The listing builds one solid part. Answer for the finished solid, in the listing's coordinates (mm). A direction names the side the tool comes from. Give positions to 0.01 mm unless a question says otherwise; leave off trailing zeros. Order: outer loops, then holes, each group sorted by start corner. A loop starts at its lowest first (then second) coordinate and runs counter-clockwise, first axis right, second up. Notation, with made-up numbers: (50, -3) - (82, -3) arc R36 ccw to (82, 31) - close; hole circle Ø4 at (89, 12.5). An arc over 180 degrees is marked (long way). Answer as a JSON object with one key per item and string values. Group by question number.
Q1. For faces 1 (the face through (-5.86, 93.18, -11.4)), 2 (the face through (-6.007, 48.669, -10.924)), 3 (the face through (11, 62.5, -30)), determine the directions among +Z, -Z, +X, -X, +Y, -Y from which every point of the face is accessible in a straight line to the end or side of a thin tool.
Q2. A cutting plane is placed at A-A, the plane y = 65. Give the vertices of the cut face in (x, z).
Q3. A cutting plane is placed at B-B, the plane y = 24. Give the vertices of the cut face in (x, z), and give its area (3 significant figures).
Q4. The mould has two halves that part along X. Classify faces 4 (the face through (18.2, 55, -20.1)), 5 (the face through (-5.86, -2.88, -11.4)), 6 (the face through (13.78, 124.33, -23.65)), 7 (the face through (-0.46, 8.52, -40.49)): released by +X, released by -X, zero draft, split by the parting line, or undercut.
Q5. Given pin 1 (3 mm diameter, centred on y = 87, z = -32, fed in from +X); pin 2 (4 mm diameter, centred on y = 43, z = -24.5, fed in from +X); pin 3 (2 mm diameter, centred on x = 13.86, z = -38, fed in from +Y), each flat-ended and moving along its own axis, determine where each tip first touches the part or whether it passes through.
Q6. Consider line 1 (X direction, y = 127.75, z = -46); line 2 (X direction, y = -2, z = -30); line 3 (X direction, y = 121.25, z = -22). Determine where each line is inside the solid, lowest interval first.
from build123d import *

# Parameters (mm, degrees)
SKETCH6_W                     = 2.15
SKETCH6_H                     = 180.5
M4_CLEARANCE_HOLE2_AT_2_COUNT = 2
M4_CLEARANCE_HOLE2_AT_2_PITCH = 16
M4_CLEARANCE_HOLE2_AT_3_COUNT = 2
M4_CLEARANCE_HOLE2_AT_3_PITCH = 27.712812921
M4_CLEARANCE_HOLE2_AT_4_COUNT = 2
M4_CLEARANCE_HOLE2_AT_4_PITCH = 32
M4_CLEARANCE_HOLE2_AT_5_COUNT = 2
M4_CLEARANCE_HOLE2_AT_5_PITCH = 27.712812921
M4_CLEARANCE_HOLE2_AT_6_COUNT = 2
M4_CLEARANCE_HOLE2_AT_6_PITCH = 16
M4_TAPPED_HOLE1_AT_2_COUNT    = 2
M4_TAPPED_HOLE1_AT_2_PITCH    = 16
M4_TAPPED_HOLE1_AT_3_COUNT    = 2
M4_TAPPED_HOLE1_AT_3_PITCH    = 27.712812921
M4_TAPPED_HOLE1_AT_4_COUNT    = 2
M4_TAPPED_HOLE1_AT_4_PITCH    = 16
M4_TAPPED_HOLE1_AT_5_COUNT    = 2
M4_TAPPED_HOLE1_AT_5_PITCH    = 27.712812921
M4_TAPPED_HOLE1_AT_6_COUNT    = 2
M4_TAPPED_HOLE1_AT_6_PITCH    = 32
SKETCH16_W                    = 1.65
SKETCH16_H                    = 19.5
SKETCH16_AT_POINT_2_W         = 1.65
SKETCH16_AT_POINT_2_H         = 19.5
SKETCH16_AT_POINT_3_W         = 1.65
SKETCH16_AT_POINT_3_H         = 19.5
SKETCH16_AT_POINT_4_W         = 1.65
SKETCH16_AT_POINT_4_H         = 19.5
SKETCH16_AT_POINT_5_W         = 1.65
SKETCH16_AT_POINT_5_H         = 19.5
SKETCH16_AT_POINT_6_W         = 1.65
SKETCH16_AT_POINT_6_H         = 19.5
CHAMFER1_SIZE                 = 0.6
FILLET1_R                     = 0.5
FILLET2_R                     = 0.4
CHAMFER2_SIZE                 = 0.5


with BuildPart() as part:
    # Sketch1 → Revolve1 (revolve)
    with BuildSketch(Plane(origin=(0, 0, 0), x_dir=(0, 0, -1), z_dir=(1, 0, 0)), mode=Mode.PRIVATE) as revolve1_sk:
        Polygon((50, 130), (50, 117), (49.5, 117), (49.5, 70), (50, 70), (50, 58), (52.5, 58), (52.5, 55), (50, 55), (50, 42.5), (49.5, 42.5), (49.5, -47), (40.5, -47), (40.5, 62.5), (42, 62.5), (42, 130), align=None)
    revolve(revolve1_sk.sketch.rotate(Axis((0, 145.844079722, -30), (0, -1, 0)), 180), axis=Axis((0, 145.844079722, -30), (0, -1, 0)))

    # Sketch12 → M4 Tapped Hole1 (revolve, cut)
    with BuildSketch(Plane(origin=(0, 130, -46), x_dir=(0, 0, 1), z_dir=(1, 0, 0))):
        Polygon((0, 0), (0, 12.491420021), (1.65, 11.5), (1.65, 0), align=None)
    m4_tapped_hole1 = revolve(axis=Axis((0, 136.35, -46), (0, -1, 0)), mode=Mode.SUBTRACT)

    # M4 Tapped Hole1 at 2: M4 Tapped Hole1 ×2
    with Locations(*[Vector(0.8660254037844387, 0, 0.5000000000000001) * (i * M4_TAPPED_HOLE1_AT_2_PITCH) for i in range(1, M4_TAPPED_HOLE1_AT_2_COUNT)]):
        add(m4_tapped_hole1, mode=Mode.SUBTRACT)

    # M4 Tapped Hole1 at 3: M4 Tapped Hole1 ×2
    with Locations(*[Vector(0.5000000000000002, 0, 0.8660254037844386) * (i * M4_TAPPED_HOLE1_AT_3_PITCH) for i in range(1, M4_TAPPED_HOLE1_AT_3_COUNT)]):
        add(m4_tapped_hole1, mode=Mode.SUBTRACT)

    # M4 Tapped Hole1 at 4: M4 Tapped Hole1 ×2
    with Locations(*[Vector(-0.8660254037844387, 0, 0.5000000000000001) * (i * M4_TAPPED_HOLE1_AT_4_PITCH) for i in range(1, M4_TAPPED_HOLE1_AT_4_COUNT)]):
        add(m4_tapped_hole1, mode=Mode.SUBTRACT)

    # M4 Tapped Hole1 at 5: M4 Tapped Hole1 ×2
    with Locations(*[Vector(-0.4999999999999997, 0, 0.8660254037844388) * (i * M4_TAPPED_HOLE1_AT_5_PITCH) for i in range(1, M4_TAPPED_HOLE1_AT_5_COUNT)]):
        add(m4_tapped_hole1, mode=Mode.SUBTRACT)

    # M4 Tapped Hole1 at 6: M4 Tapped Hole1 ×2
    with Locations(*[(0, 0, i * M4_TAPPED_HOLE1_AT_6_PITCH) for i in range(1, M4_TAPPED_HOLE1_AT_6_COUNT)]):
        add(m4_tapped_hole1, mode=Mode.SUBTRACT)

    # Sketch16 → M4 Tapped Hole2 (revolve, cut)
    with BuildSketch(Plane(origin=(12.534358389, 35.5, -15.062133359), x_dir=(0.7660444431189759, 0, -0.642787609686542), z_dir=(0, 1, 0))):
        with Locations((0.825, 9.75)):
            Rectangle(SKETCH16_W, SKETCH16_H)
    revolve(axis=Axis((16.61605971, 35.5, -10.197751145), (-0.6427876096865419, 0, -0.7660444431189758)), mode=Mode.SUBTRACT)

    # Sketch16 at point 2 (carried to point 2, square into its face) → M4 Tapped Hole2 at 2 (revolve, cut)
    with BuildSketch(Plane(origin=(12.534358389, 0, -15.062133359), x_dir=(0.766044068, 0, -0.642788057), z_dir=(0, 1, 0))):
        with Locations((0.825, 9.75)):
            Rectangle(SKETCH16_AT_POINT_2_W, SKETCH16_AT_POINT_2_H)
    revolve(axis=Axis((16.61606255, 0, -10.197753528), (-0.642788057, 0, -0.766044068)), mode=Mode.SUBTRACT)

    # Sketch16 at point 3 (carried to point 3, square into its face) → M4 Tapped Hole2 at 3 (revolve, cut)
    with BuildSketch(Plane(origin=(12.534358389, -35.5, -15.062133359), x_dir=(0.766044068, 0, -0.642788057), z_dir=(0, 1, 0))):
        with Locations((0.825, 9.75)):
            Rectangle(SKETCH16_AT_POINT_3_W, SKETCH16_AT_POINT_3_H)
    revolve(axis=Axis((16.61606255, -35.5, -10.197753528), (-0.642788057, 0, -0.766044068)), mode=Mode.SUBTRACT)

    # Sketch16 at point 4 (carried to point 4, square into its face) → M4 Tapped Hole2 at 4 (revolve, cut)
    with BuildSketch(Plane(origin=(-12.534358389, -35.5, -15.062133359), x_dir=(0.766044068, 0, 0.642788057), z_dir=(0, 1, 0))):
        with Locations((0.825, 9.75)):
            Rectangle(SKETCH16_AT_POINT_4_W, SKETCH16_AT_POINT_4_H)
    revolve(axis=Axis((-16.61606255, -35.5, -10.197753528), (0.642788057, 0, -0.766044068)), mode=Mode.SUBTRACT)

    # Sketch16 at point 5 (carried to point 5, square into its face) → M4 Tapped Hole2 at 5 (revolve, cut)
    with BuildSketch(Plane(origin=(-12.534358389, 0, -15.062133359), x_dir=(0.766044068, 0, 0.642788057), z_dir=(0, 1, 0))):
        with Locations((0.825, 9.75)):
            Rectangle(SKETCH16_AT_POINT_5_W, SKETCH16_AT_POINT_5_H)
    revolve(axis=Axis((-16.61606255, 0, -10.197753528), (0.642788057, 0, -0.766044068)), mode=Mode.SUBTRACT)

    # Sketch16 at point 6 (carried to point 6, square into its face) → M4 Tapped Hole2 at 6 (revolve, cut)
    with BuildSketch(Plane(origin=(-12.534358389, 35.5, -15.062133359), x_dir=(0.766044068, 0, 0.642788057), z_dir=(0, 1, 0))):
        with Locations((0.825, 9.75)):
            Rectangle(SKETCH16_AT_POINT_6_W, SKETCH16_AT_POINT_6_H)
    revolve(axis=Axis((-16.61606255, 35.5, -10.197753528), (0.642788057, 0, -0.766044068)), mode=Mode.SUBTRACT)

    # Chamfer1
    chamfer1_edges = [part.edges().sort_by_distance(p)[0] for p in [
        (0, 130, -50),
    ]]
    chamfer(chamfer1_edges, length=CHAMFER1_SIZE)

    # Fillet1
    fillet1_edges = [part.edges().sort_by_distance(p)[0] for p in [
        (0, 58, -50),
        (0, 55, -50),
    ]]
    fillet(fillet1_edges, radius=FILLET1_R)

    # Chamfer2
    chamfer2_edges = [part.edges().sort_by_distance(p)[0] for p in [
        (0, 42.5, -50),
        (0, 117, -49.5),
        (0, 70, -49.5),
    ]]
    chamfer(chamfer2_edges, length=CHAMFER2_SIZE - 0.0001)  # a hair under: the kernel refuses the full size


with BuildPart() as body_2:
    # Sketch2 → Revolve2 (revolve)
    with BuildSketch(Plane(origin=(0, 0, 0), x_dir=(0, 0, -1), z_dir=(1, 0, 0)), mode=Mode.PRIVATE) as revolve2_sk:
        Polygon((42, 133.5), (52.5, 133.5), (52.5, 129), (50, 129), (50, 130.5), (42, 130.5), align=None)
    revolve(revolve2_sk.sketch.rotate(Axis((0, 145.844079722, -30), (0, -1, 0)), 180), axis=Axis((0, 145.844079722, -30), (0, -1, 0)))

    # Sketch6 → M4 Clearance Hole2 (revolve, cut)
    with BuildSketch(Plane(origin=(-13.856406461, 133.5, -38), x_dir=(0, 0, 1), z_dir=(1, 0, 0))):
        with Locations((1.075, 90.25)):
            Rectangle(SKETCH6_W, SKETCH6_H)
    m4_clearance_hole2 = revolve(axis=Axis((-13.856406461, 139.85, -38), (0, -1, 0)), mode=Mode.SUBTRACT)

    # M4 Clearance Hole2 at 2: M4 Clearance Hole2 ×2
    with Locations(*[Vector(0.8660254037844387, 0, -0.5000000000000001) * (i * M4_CLEARANCE_HOLE2_AT_2_PITCH) for i in range(1, M4_CLEARANCE_HOLE2_AT_2_COUNT)]):
        add(m4_clearance_hole2, mode=Mode.SUBTRACT)

    # M4 Clearance Hole2 at 3: M4 Clearance Hole2 ×2
    with Locations(*[(i * M4_CLEARANCE_HOLE2_AT_3_PITCH, 0, 0) for i in range(1, M4_CLEARANCE_HOLE2_AT_3_COUNT)]):
        add(m4_clearance_hole2, mode=Mode.SUBTRACT)

    # M4 Clearance Hole2 at 4: M4 Clearance Hole2 ×2
    with Locations(*[Vector(0.8660254037844387, 0, 0.49999999999999994) * (i * M4_CLEARANCE_HOLE2_AT_4_PITCH) for i in range(1, M4_CLEARANCE_HOLE2_AT_4_COUNT)]):
        add(m4_clearance_hole2, mode=Mode.SUBTRACT)

    # M4 Clearance Hole2 at 5: M4 Clearance Hole2 ×2
    with Locations(*[Vector(0.5000000000000001, 0, 0.8660254037844387) * (i * M4_CLEARANCE_HOLE2_AT_5_PITCH) for i in range(1, M4_CLEARANCE_HOLE2_AT_5_COUNT)]):
        add(m4_clearance_hole2, mode=Mode.SUBTRACT)

    # M4 Clearance Hole2 at 6: M4 Clearance Hole2 ×2
    with Locations(*[(0, 0, i * M4_CLEARANCE_HOLE2_AT_6_PITCH) for i in range(1, M4_CLEARANCE_HOLE2_AT_6_COUNT)]):
        add(m4_clearance_hole2, mode=Mode.SUBTRACT)

    # Fillet2
    fillet2_edges = [body_2.edges().sort_by_distance(p)[0] for p in [
        (0, 130.5, -50),
    ]]
    fillet(fillet2_edges, radius=FILLET2_R)


solid = part.part
Reply:
{
 "1": {"face 1": "none", "face 2": "-Y", "face 3": "+Y"},
 "2": {"outline": "circle Ø40 at (0, -30); hole circle Ø24 at (0, -30)"},
 "3": {"outline": "circle Ø39 at (0, -30); hole circle Ø21 at (0, -30)", "area": "848 mm^2"},
 "4": {"face 4": "zero draft", "face 5": "split by the parting line", "face 6": "undercut", "face 7": "undercut"},
 "5": {"pin 1": "stops at x = 19.49", "pin 2": "stops at x = 19.69", "pin 3": "stops at y = 118.11"},
 "6": {"line 1": "x = -12 to -1.65, 1.65 to 12", "line 2": "x = -19.5 to -10.5, 10.5 to 19.5", "line 3": "x = -18.33 to -15.51, -12.21 to -8.94, 8.94 to 12.21, 15.51 to 18.33"}
}
